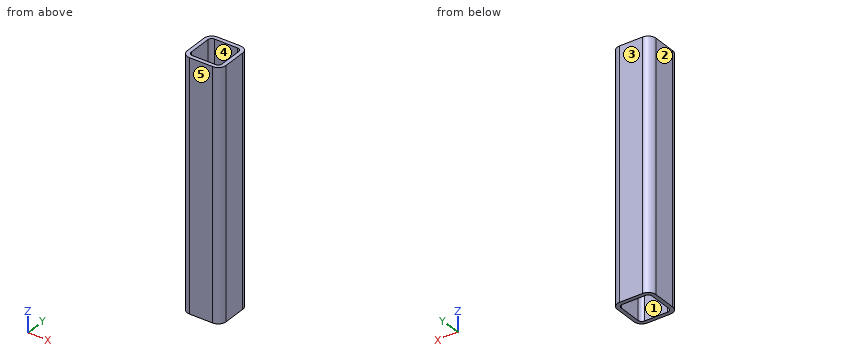
Autodesk Inventor part; units mm, degrees
ref_plane "Start Plane" through (0, 0, 15) normal (0, 0, 1) x (1, 0, 0)
ref_plane "End Plane" through (0, 0, 207) normal (0, 0, 1) x (1, 0, 0)
ref_plane "Work Plane4" through (-9, -370, 15) normal (0, 0, -1) x (-1, 0, 0)
ref_plane "Start Plane" through (0, 0, 15) normal (0, 0, 1) x (1, 0, 0)
ref_plane "End Plane" through (0, 0, 207) normal (0, 0, 1) x (1, 0, 0)
sketch "Sketch" plane through (0, 0, 0) normal (0, 0, 1) x (1, 0, 0)
  line L0 (-15, -9) -> (-15, 9)
  line L1 (-9, 15) -> (9, 15)
  line L2 (15, 9) -> (15, -9)
  line L3 (9, -15) -> (-9, -15)
  arc A0 (-15, -9) -> (-9, -15) centre (-9, -9) ccw
  arc A1 (-9, 15) -> (-15, 9) centre (-9, 9) ccw
  arc A2 (15, 9) -> (9, 15) centre (9, 9) ccw
  arc A3 (9, -15) -> (15, -9) centre (9, -9) ccw
  arc A4 (-9, 12) -> (-12, 9) centre (-9, 9) ccw
  line L4 (-9, 12) -> (9, 12)
  arc A5 (12, 9) -> (9, 12) centre (9, 9) ccw
  line L5 (12, 9) -> (12, -9)
  arc A6 (9, -12) -> (12, -9) centre (9, -9) ccw
  line L6 (9, -12) -> (-9, -12)
  arc A7 (-12, -9) -> (-9, -12) centre (-9, -9) ccw
  line L7 (-12, -9) -> (-12, 9)
  line L8 (0, 22.7397) -> (0, -22.7397) construction
  line L9 (-22.7397, 0) -> (22.7397, 0) construction
  dimension "d7" = 6
  dimension "d10" = 30
  dimension "d11" = 30
  dimension "d12" = 3
  dimension "d15" = 15
  dimension "d16" = 15
extrude "Body" add sketch "Sketch" along normal up to surface (192 mm away) from surface at 15
sketch "Sketch3" plane through (0, 0, 0) normal (0, 0, 1) x (1, 0, 0)
  line L0 (0, 0) -> (10, 0)
ref_plane "Work Plane3" through (0, 0, 0) normal (0, -1, 0) x (1, 0, 0)
ref_plane "Work Plane4" through (-9, -370, 15) normal (0, 0, -1) x (-1, 0, 0)
split "Split1" plane through (-9, -370, 15) removes the side toward (0, 0, -1)
ref_plane "Work Plane5" through (-9, 130, 207) normal (0, 0, 1) x (1, 0, 0)
split "Split2" plane through (-9, 130, 207) removes the side toward (0, 0, 1)
sketch "Sketch4" plane through (0, 0, 0) normal (0, -1, 0) x (1, 0, 0)
  line L0 (-2, 15) -> (12, 15)
  line L1 (-2, 207) -> (12, 207)
  dimension "d18" = 192
equation "\"d7\" = G_IR"
equation "\"d10\" = G_H"
equation "\"d11\" = G_W"
equation "\"d12\" = G_T"
equation "\"d15\" = 0.5 * d10"
equation "\"d16\" = 0.5 * d11"
equation "\"d3\" = G_L"
equation "\"G_W\" = 30"
equation "\"G_H\" = 30"
equation "\"G_T\" = 3"
equation "\"G_IR\" = 6"
equation "\"G_L\" = d18"
equation "\"G_OFFSET_START\" = -15"
equation "\"G_OFFSET_END\" = -15"
equation "\"d13\" = -G_OFFSET_START"
equation "\"d14\" = G_OFFSET_END + B_L"
equation "\"B_L\" = 222"
properties part number "DIN EN 10219-2 - 30 x 30 x 3  - 192" material "Steel, Mild"
The model under review builds one solid part; all positions refer to its coordinate system, in mm. Face numbers are marked on the shaded views. A direction names the side the tool comes from. Round coordinates to 2 decimals unless told otherwise and drop trailing zeros. Loops run counter-clockwise (first coordinate to the right, second up) from the corner with the lowest first, then second, coordinate; pieces in that order, holes last. Notation, with made-up numbers: (38, 11) -> (71, 11) arc R19 cw to (71, 33) -> close; hole circle Ø10 at (19, 21.5). An arc over 180 degrees is marked (long way). Answer as a JSON object with one key per item and string values. Group by question number.
1) For the marked faces 4 and 5, list the 3-axis set-ups (+Z, -Z, +X, -X, +Y, -Y) from which the entire face can be reached by the end or side of a thin tool; tool diameter is ignored.
2) For line 1 (X direction, y = -3, z = 64.5); line 2 (Y direction, x = 11.5, z = 109), list the stretches that pass through material, from the lowest coordinate up. Write a range as [from, to].
3) We need section A-A on x = 3.25. Write out the cut boundary in (y, z), then the cut area to 3 significant figures.
4) Mouldability with a two-part tool opening along Y and no side actions: class the marked faces 1, 2 and 3 as released by +Y, released by -Y, zero draft, split by the parting line, or undercut.
5) For pin 1 Ø1.5 at (x, z) = (10.5, 102.5) entering from -Y, flat-tipped, find the tip position at first contact; note if it passes through.
6) We need section B-B on z = 149.5. Write out the cut boundary in (x, y), then the cut area to 3 significant figures.
Result set:
{
 "1": {"face 4": "+Z, -Z", "face 5": "+Z, -Z, +X, -X, -Y"},
 "2": {"line 1": "[-15, -12], [12, 15]", "line 2": "[-14.45, -10.66], [10.66, 14.45]"},
 "3": {"outline": "(-15, 15) -> (-12, 15) -> (-12, 207) -> (-15, 207) -> close; (12, 15) -> (15, 15) -> (15, 207) -> (12, 207) -> close", "area": "1,150 mm²"},
 "4": {"face 1": "undercut", "face 2": "zero draft", "face 3": "released by +Y"},
 "5": {"pin 1": "y = -14.95"},
 "6": {"outline": "(-15, -9) arc R6 ccw to (-9, -15) -> (9, -15) arc R6 ccw to (15, -9) -> (15, 9) arc R6 ccw to (9, 15) -> (-9, 15) arc R6 ccw to (-15, 9) -> close; hole (-12, -9) arc R3 ccw to (-9, -12) -> (9, -12) arc R3 ccw to (12, -9) -> (12, 9) arc R3 ccw to (9, 12) -> (-9, 12) arc R3 ccw to (-12, 9) -> close", "area": "301 mm²"}
}
